Autodesk Inventor part; units mm, degrees
ref_plane "YZ Plane" through (0, 0, 0) normal (1, 0, 0) x (0, 1, 0)
ref_plane "XZ Plane" through (0, 0, 0) normal (0, 1, 0) x (-1, 0, 0)
ref_plane "XY Plane" through (0, 0, 0) normal (0, 0, 1) x (1, 0, 0)
sketch "Sketch1" plane through (0, 0, 0) normal (1, 0, 0) x (0, 1, 0)
  line L0 (0, 0) -> (63.5, 0)
  line L1 (63.5, 0) -> (63.5, 44.45)
  line L2 (0, 44.45) -> (0, 0)
  line L3 (31.75, 139.6202) -> (31.75, -24.2766) construction
  arc A0 (53.7441, 111.6025) -> (9.7559, 111.6025) centre (31.75, 108.4072) ccw
  line L4 (63.5, 44.45) -> (53.7441, 111.6025)
  line L5 (0, 44.45) -> (9.7559, 111.6025)
  line L6 (0, 22.225) -> (-15.9644, 22.225)
  point P0 (31.75, 25.908)
  dimension "d0" = 63.5
  dimension "d1" = 44.45
  dimension "d3" = 31.75
  dimension "d5" = 44.45
  dimension "d21" = 82.4992
  dimension "d22" = 63.9572
  dimension "d40" = 25.908
extrude "Extrusion1" add sketch "Sketch1" along normal blind 2.286
hole "Hole2" at (0, 31.75, 108.4072) at (0, 31.75, 25.908) direction (1, 0, 0) diameter 28.575 end through all
sketch "Sketch2" plane through (2.286, 0, 0) normal (1, 0, 0) x (0, 0, -1)
  line L0 (0, 63.5) -> (-44.45, 63.5)
  line L1 (-12.7, -16.6387) -> (-12.7, 68.9005) construction
  line L2 (0, 0) -> (0, 63.5) construction
  circle A0 centre (-25.908, 31.75) radius 14.2875
  circle A1 centre (-25.908, 31.75) radius 22.0437
  circle A2 centre (-6.35, 57.15) radius 4.5847
  line L3 (-0.8507, 57.15) -> (-3.6004, 52.3875)
  line L4 (-3.6004, 52.3875) -> (-9.0996, 52.3875)
  line L5 (-9.0996, 52.3875) -> (-11.8493, 57.15)
  line L6 (-11.8493, 57.15) -> (-9.0996, 61.9125)
  line L7 (-9.0996, 61.9125) -> (-3.6004, 61.9125)
  line L8 (-3.6004, 61.9125) -> (-0.8507, 57.15)
  circle A3 centre (-34.925, 57.15) radius 4.5847
  line L9 (-29.631, 57.15) -> (-32.278, 52.5653)
  line L10 (-32.278, 52.5653) -> (-37.572, 52.5653)
  line L11 (-37.572, 52.5653) -> (-40.219, 57.15)
  line L12 (-40.219, 57.15) -> (-37.572, 61.7347)
  line L13 (-37.572, 61.7347) -> (-32.278, 61.7347)
  line L14 (-32.278, 61.7347) -> (-29.631, 57.15)
  point P0 (-6.35, 6.35)
  point P1 (-34.925, 6.35)
  dimension "d33" = 9.1694
  dimension "d35" = 9.525
  dimension "d37" = 25.4
  dimension "d39" = 25.4
  dimension "d41" = 9.525
  dimension "d42" = 38.1
hole "Hole1" at (2.286, 57.15, 34.925) at (2.286, 57.15, 6.35) at (2.286, 6.35, 34.925) at (2.286, 6.35, 6.35) direction (-1, 0, 0) diameter 5.1054 end through all
equation "\"d3\" = 0.5 * d0"
properties part number "CAR_041_KickerGusset" material "Aluminum 6061"
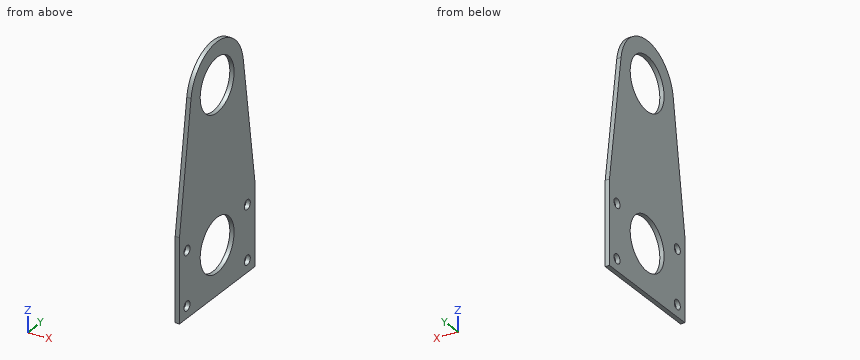
Geometry check sheet. Reference: the model listing, model coordinates, mm. Round coordinates to 2 decimals unless told otherwise and drop trailing zeros. Loops run counter-clockwise (first coordinate to the right, second up) from the corner with the lowest first, then second, coordinate; pieces in that order, holes last. Notation, with made-up numbers: (53, 22) - (84, 22) arc R20 cw to (84, 36) - close; hole circle Ø10 at (67, -22.5). An arc over 180 degrees is marked (long way). Write each question's results on one line, items separated by ' | '. Start each with the question number.
Q1. Cross-section at B-B on x = 1.9. State how many separate pieces and enclosed holes the cut face has, and give its area (3 significant figures).
Q2. Gauge pin test, flat end, axial feed: P1, Ø6.5, axis at y = 57.15, z = 34.925, coming from the -X side. Record the tip position at first contact, or that the pin passes through.
Q3. Cross-section at A-A on z = 6.35. Enter the section's corners in (x, y).
Q4. Cross-section at D-D on y = 6.35. Enter the section's corners in (x, z).
Q5. Thickness scan on line 1 (Z direction, x = 0.5, y = 31.75); line 2 (Y direction, x = 1.6, z = 6.35); line 3 (Z direction, x = 1.7, y = 44). Record the ranges inside material, lowest first. Write a range as [from, to].
Q6. Cross-section at C-C on z = 119.5. Enter the section's corners in (x, y).
Answers below:
1) separate pieces: 1 | enclosed holes: 6 | area: 5,700 mm²
2) P1: stops at x = 0
3) outline: (0, 0) - (2.29, 0) - (2.29, 3.8) - (0, 3.8) - close; (0, 8.9) - (2.29, 8.9) - (2.29, 54.6) - (0, 54.6) - close; (0, 59.7) - (2.29, 59.7) - (2.29, 63.5) - (0, 63.5) - close
4) outline: (0, 0) - (2.29, 0) - (2.29, 3.8) - (0, 3.8) - close; (0, 8.9) - (2.29, 8.9) - (2.29, 32.37) - (0, 32.37) - close; (0, 37.48) - (2.29, 37.48) - (2.29, 88.16) - (0, 88.16) - close
5) line 1: z = [0, 11.62], [40.2, 94.12], [122.69, 130.63] | line 2: y = [0, 3.8], [8.9, 54.6], [59.7, 63.5] | line 3: z = [0, 18.55], [33.26, 101.05], [115.76, 126.95]
6) outline: (0, 12.49) - (2.29, 12.49) - (2.29, 22.75) - (0, 22.75) - close; (0, 40.75) - (2.29, 40.75) - (2.29, 51.01) - (0, 51.01) - close
